Geometry: final body of the model. Coordinates: model frame, mm. Face numbers are marked on the shaded views. A direction names the side the tool comes from. Coordinates: 2 decimals unless noted, no trailing zeros. Write each loop counter-clockwise with the first axis right and the second up, starting at its lowest first coordinate (ties: lowest second). Pieces come first, ordered by that corner, then holes. Notation, with made-up numbers: (-34.75, 16.5) - (3.25, 16.5) arc R31 ccw to (3.25, 50.5) - close; hole circle Ø8 at (-9, 46.25). An arc over 180 degrees is marked (long way). Put each result on its own line as item: value.
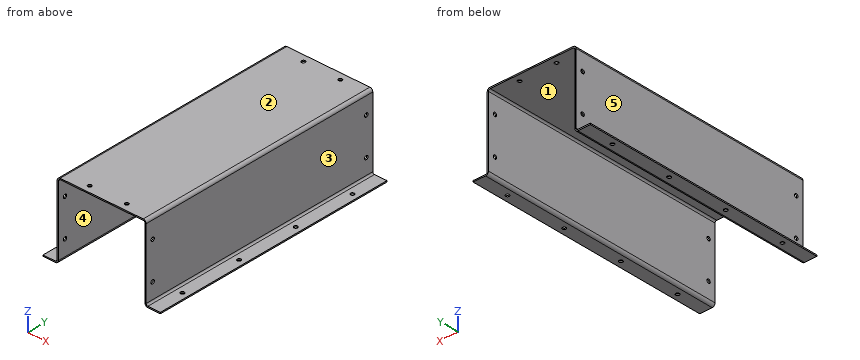
Autodesk Inventor part; units mm, degrees
ref_plane "YZ Plane" through (0, 0, 0) normal (1, 0, 0) x (0, 1, 0)
ref_plane "XZ Plane" through (0, 0, 0) normal (0, 1, 0) x (-1, 0, 0)
ref_plane "XY Plane" through (0, 0, 0) normal (0, 0, 1) x (1, 0, 0)
sketch "Sketch1" plane through (0, 0, 0) normal (0, 0, 1) x (1, 0, 0)
  line L0 (-70, 200) -> (70, 200)
  line L1 (70, 200) -> (70, -200)
  line L2 (70, -200) -> (-70, -200)
  line L3 (-70, -200) -> (-70, 200)
  line L4 (-70, 200) -> (70, -200) construction
  point P0 (0, 0)
  point P1 (0, 0)
  dimension "d0" = 140
  dimension "d1" = 400
extrude "Plate1" add sketch "Sketch1" along normal blind 2
sketch "Sketch2" plane through (72, -200, 2) normal (-1, 0, 0) x (0, -1, 0)
  line L0 (-400, 0) -> (0, 0)
  line L1 (0, 0) -> (0, -120)
  line L2 (0, -120) -> (-400, -120)
  line L3 (-400, -120) -> (-400, 0)
edge flange "Flange1" height 120 angle 90 thickness 2 bend radius 2.75 thickness toward (-1, 0, 0) relief round relief width 2 relief depth 1 edges at (70, 0, 0) wall of the first edge with corners at (72, 200, 2) (72, -200, 2) (72, -200, -118) (72, 200, -118)
bend "Bend1"
corner "Corner1"
sketch "Sketch3" plane through (-72, 200, 2) normal (1, 0, 0) x (0, 1, 0)
  line L0 (-400, 0) -> (0, 0)
  line L1 (0, 0) -> (0, -120)
  line L2 (0, -120) -> (-400, -120)
  line L3 (-400, -120) -> (-400, 0)
edge flange "Flange2" height 120 angle 90 thickness 2 bend radius 2.75 thickness toward (1, 0, 0) relief round relief width 2 relief depth 1 edges at (-70, 0, 0) wall of the first edge with corners at (-72, -200, 2) (-72, 200, 2) (-72, 200, -118) (-72, -200, -118)
bend "Bend2"
corner "Corner2"
sketch "Sketch4" plane through (70, 200, -120) normal (0, 0, 1) x (1, 0, 0)
  line L0 (0, -400) -> (0, 0)
  line L1 (0, 0) -> (25, 0)
  line L2 (25, 0) -> (25, -400)
  line L3 (25, -400) -> (0, -400)
edge flange "Flange3" height 25 angle 90 thickness 2 bend radius 2.75 thickness toward (0, 0, 1) relief round relief width 2 relief depth 1 edges at (72, 0, -118) wall of the first edge with corners at (70, -200, -120) (70, 200, -120) (95, 200, -120) (95, -200, -120)
bend "Bend3"
corner "Corner3"
sketch "Sketch5" plane through (-70, -200, -120) normal (0, 0, 1) x (1, 0, 0)
  line L0 (0, 400) -> (0, 0)
  line L1 (0, 0) -> (-25, 0)
  line L2 (-25, 0) -> (-25, 400)
  line L3 (-25, 400) -> (0, 400)
edge flange "Flange4" height 25 angle 90 thickness 2 bend radius 2.75 thickness toward (0, 0, 1) relief round relief width 2 relief depth 1 edges at (-72, 0, -118) wall of the first edge with corners at (-70, 200, -120) (-70, -200, -120) (-95, -200, -120) (-95, 200, -120)
bend "Bend4"
corner "Corner4"
sketch "Sketch6" plane through (95, -200, -118) normal (0, 0, 1) x (1, 0, 0)
  circle A0 centre (-10.125, 350) radius 3
  line L0 (-20.25, 400) -> (0, 400)
  point P0 (-95, 200)
  point P1 (-10.125, 400)
  dimension "d43" = 6
  dimension "d44" = 50
extrude "Extrusion1" cut sketch "Sketch6" against normal through all
pattern_linear "Rectangular Pattern2" count 4 spacing 100 along (0, -1, 0) count 2 spacing 169.75 along (-1, 0, 0) of "Extrusion1"
sketch "Sketch8" plane through (72, -200, -2.75) normal (1, 0, 0) x (0, 0, -1)
  line L0 (0, 400) -> (112.5, 400)
  line L1 (117.25, 0) -> (117.25, 400)
  circle A0 centre (87.25, 388.5) radius 3
  circle A1 centre (27.25, 388.5) radius 3
  point P0 (-2.75, 200)
  dimension "d68" = 6
  dimension "d69" = 60
  dimension "d78" = 30
  dimension "d79" = 11.5
extrude "Extrusion3" cut sketch "Sketch8" against normal through all
sketch "Sketch9" plane through (0, 0, 2) normal (0, 0, 1) x (1, 0, 0)
  circle A0 centre (-29.95, 188.5) radius 3
  line L0 (-67.25, 200) -> (67.25, 200)
  line L1 (-67.25, 200) -> (-67.25, -200)
  circle A1 centre (30.05, 188.5) radius 3
  point P0 (0, 0)
  point P1 (67.25, 200)
  dimension "d72" = 6
  dimension "d73" = 11.5
  dimension "d74" = 37.3
  dimension "d80" = 60
extrude "Extrusion4" cut sketch "Sketch9" against normal through all
mirror "Mirror2" about plane through (0, 0, 0) normal (0, 1, 0) of "Extrusion3", "Extrusion4"
equation "\"d0\" = Ширина_крепления_корпуса"
equation "\"d1\" = Длина_базовой_пластины"
equation "\"d69\" = 0.5 * Длина_крепления_корпуса"
equation "\"d2\" = Thickness"
equation "\"d3\" = BendReliefWidth"
equation "\"d4\" = BendReliefDepth"
equation "\"d5\" = MinimumRemnant"
equation "\"d6\" = TransitionRadius"
equation "\"d7\" = Длина_крепления_корпуса"
equation "\"d9\" = BendRadius"
equation "\"d10\" = CornerReliefSize"
equation "\"d11\" = GapSize"
equation "\"d12\" = JacobiRadiusSize"
equation "\"d13\" = BendReliefWidth"
equation "\"d14\" = BendReliefDepth"
equation "\"d15\" = MinimumRemnant"
equation "\"d16\" = TransitionRadius"
equation "\"d17\" = Длина_крепления_корпуса"
equation "\"d19\" = BendRadius"
equation "\"d20\" = CornerReliefSize"
equation "\"d21\" = GapSize"
equation "\"d22\" = JacobiRadiusSize"
equation "\"d23\" = BendReliefWidth"
equation "\"d24\" = BendReliefDepth"
equation "\"d25\" = MinimumRemnant"
equation "\"d26\" = TransitionRadius"
equation "\"d29\" = BendRadius"
equation "\"d30\" = CornerReliefSize"
equation "\"d31\" = GapSize"
equation "\"d32\" = JacobiRadiusSize"
equation "\"d33\" = BendReliefWidth"
equation "\"d34\" = BendReliefDepth"
equation "\"d35\" = MinimumRemnant"
equation "\"d36\" = TransitionRadius"
equation "\"d39\" = BendRadius"
equation "\"d40\" = CornerReliefSize"
equation "\"d41\" = GapSize"
equation "\"d42\" = JacobiRadiusSize"
equation "\"BendReliefWidth\" = Thickness"
equation "\"BendReliefDepth\" = 0.5 * Thickness"
equation "\"CornerReliefSize\" = 4 * Thickness"
equation "\"MinimumRemnant\" = 2 * Thickness"
equation "\"TransitionRadius\" = BendRadius"
equation "\"JacobiRadiusSize\" = BendRadius"
equation "\"GapSize\" = Thickness"
properties part number "Кожух" material "Stainless Steel"
1. Mould query, pull axis X, two halves, no side actions, for the marked faces 1, 2 and 3. Classes: +X half, -X half, draft (parallel to the pull), parting line (faces both ways), or undercut.
Answer below:
face 1: undercut
face 2: draft
face 3: +X half
2. Section query C-C (x = 56.5). Return loops of the section in (y, z).
Answer below:
outline: (-200, 0) - (200, 0) - (200, 2) - (-200, 2) - close
3. Ray query, probe 1 along X at (y, z) = (62, -44); probe 2 along Y at (x, z) = (-29.95, 0.5); probe 3 along Z at (x, y) = (70.4, 188.5). Return the intervals inside material, ascending. Write a range as from..to.
Answer below:
probe 1: x = -72..-70, 70..72
probe 2: y = -200..-191.5, -185.5..185.5, 191.5..200
probe 3: z = -117.16..-93, -87..-33, -27..0.81
4. Section query B-B (y = 73). Return loops of the section in (x, z).
Answer below:
outline: (-95, -120) - (-74.75, -120) arc R4.75 ccw to (-70, -115.25) - (-70, -2.75) arc R2.75 cw to (-67.25, 0) - (67.25, 0) arc R2.75 cw to (70, -2.75) - (70, -115.25) arc R4.75 ccw to (74.75, -120) - (95, -120) - (95, -118) - (74.75, -118) arc R2.75 cw to (72, -115.25) - (72, -2.75) arc R4.75 ccw to (67.25, 2) - (-67.25, 2) arc R4.75 ccw to (-72, -2.75) - (-72, -115.25) arc R2.75 cw to (-74.75, -118) - (-95, -118) - close
5. Set-up query: the marked faces 4 and 5. Return all of +Z, -Z, +X, -X, +Y, -Y with unobstructed straight access to the full face (end or side cutting, diameter ignored); none if empty.
Answer below:
face 4: -Z, +Y, -Y
face 5: +Z, -X, +Y, -Y
6. Pin query (flat end, axial travel): pin 1 Ø10 at (x, y) = (45.5, 137) entering from -Z; pin 2 Ø3 at (y, z) = (-27.5, -18) entering from -X; pin 3 Ø12 at (y, z) = (-29.5, -75.5) entering from +X; pin 4 Ø3.5 at (y, z) = (188.5, -90) entering from -X. Return the tip coordinate at first contact, or that it passes through.
Answer below:
pin 1: stops at z = 0
pin 2: stops at x = -72
pin 3: stops at x = 72
pin 4: passes through
7. Section query A-A (z = -72.5). Return loops of the section in (x, y).
Answer below:
outline: (-72, -200) - (-70, -200) - (-70, 200) - (-72, 200) - close; (70, -200) - (72, -200) - (72, 200) - (70, 200) - close
